Verification items for this drawing (mm, ordinates from the low corner). Give positions to 0.01 mm unless a question says otherwise; leave off trailing zeros. Loops run counter-clockwise (first coordinate to the right, second up) from the corner with the lowest first, then second, coordinate; pieces in that order, holes last. Notation, with made-up numbers: (86.25, -38.5) -> (137.25, -38.5) arc R18 ccw to (137.25, -11.5) -> close; hole circle Ø1 at (7, -10). An arc over 180 degrees is marked (long way). Write item = value, one per line.
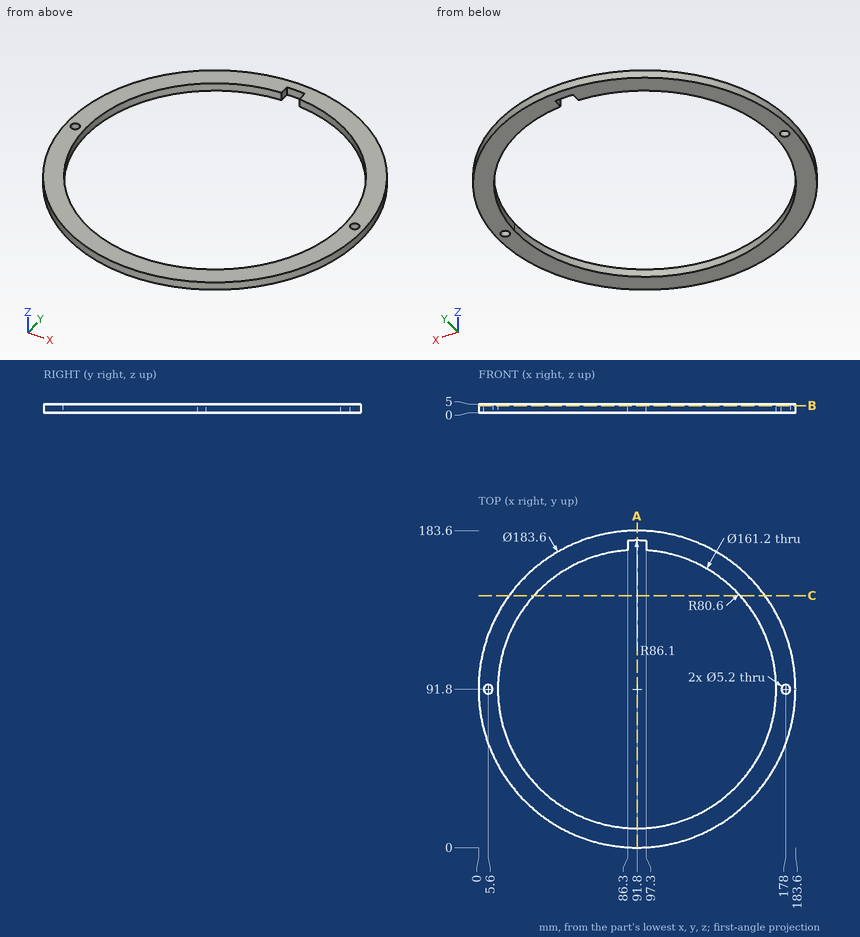
Item 1: Section check C-C, the plane y = 146. Record the cut outline in (x, z) (3 decimals).
Answer:
outline = (17.708, 0) -> (32.145, 0) -> (32.145, 5) -> (17.708, 5) -> close; (151.455, 0) -> (165.892, 0) -> (165.892, 5) -> (151.455, 5) -> close
Item 2: Section check B-B, the plane z = 4.1. Record the cut outline in (x, y), plus the area to 3 significant figures.
Answer:
outline = circle Ø183.6 at (91.8, 91.8); hole circle Ø5.2 at (5.6, 91.8); hole (86.3, 172.21) arc R80.6 ccw (long way) to (97.3, 172.21) -> (97.3, 177.72) arc R86.1 ccw to (86.3, 177.72) -> close; hole circle Ø5.2 at (178, 91.8)
area = 5,960 mm^2
Item 3: Thickness scan on L1, parallel to Y at x = 91.8, z = 2.6; L2, parallel to X at y = 94, z = 2.7; L3, parallel to Y at x = 74, z = 3.2. Record the ranges inside material, lowest first. Write a range as [from, to].
Answer:
L1 = [0, 11.2], [177.9, 183.6]
L2 = [0.03, 4.21], [6.99, 11.23], [172.37, 176.61], [179.39, 183.57]
L3 = [1.74, 13.19], [170.41, 181.86]
Item 4: Section check A-A, the plane x = 91.8. Record the cut outline in (y, z), plus the area to 3 significant figures.
Answer:
outline = (0, 0) -> (11.2, 0) -> (11.2, 5) -> (0, 5) -> close; (177.9, 0) -> (183.6, 0) -> (183.6, 5) -> (177.9, 5) -> close
area = 84.5 mm^2
Item 5: Gauge pin test, flat ends, axial feed: pin 1 (7 mm diameter, centred on x = 5.6, y = 91.8, fed in from -Z); pin 2 (1.5 mm diameter, centred on y = 174, z = 1.5, fed in from +X); pin 3 (1.5 mm diameter, centred on x = 41.5, z = 3, fed in from -Y). Record the tip position at first contact, or that the pin passes through.
Answer:
pin_1 = 0
pin_2 = 134.15
pin_3 = 14.52
